Can you work these out from the model? Positions are in its coordinate system, mm. Face numbers are marked on the shaded views. Coordinates: 2 decimals unless noted, no trailing zeros. Order: outer loops, then holes, each group sorted by start corner. A loop starts at its lowest first (then second) coordinate and runs counter-clockwise, first axis right, second up. Notation, with made-up numbers: (79.5, -9) - (134.5, -9) arc R20 ccw to (134.5, 8) - close; hole circle Ø3 at (26, -7). An arc over 180 degrees is marked (long way). Use a Markdown table: item, result. Add a question column.
(1) If I drill on L1, parallel to Y at x = 0, z = 1.9; L2, parallel to X at y = -34.5, z = 1.95; L3, parallel to Y at x = 7.75, z = 0.95, over which ranges is the centre line in solid material (lowest first)? Write a range as [from, to].
(2) I want a section at D-D (x = 5.5). List the corners of the cut face in (y, z) for me.
(3) I want a section at B-B (z = 1.35). List the corners of the cut face in (x, y) for me.
(4) I want a section at C-C (y = -24.25). List the corners of the cut face in (x, z) for me, and give its area (4 significant figures).
(5) We'd pull the mould along Y, two halves only. Please class the marked faces 1, 2, 3 and 4: pulls with the +Y half, pulls with the -Y half, needs draft (parallel to the pull), parting line crosses it, or undercut.
(6) I want a section at A-A (x = 0). List the corners of the cut face in (y, z) for me, and give its area (3 significant figures).
(7) For pin 1 Ø1.5 at (y, z) = (-5, 2.5) entering from -X, with a flat end and sliding along its axis, tell me the tip position at first contact or that it passes through.
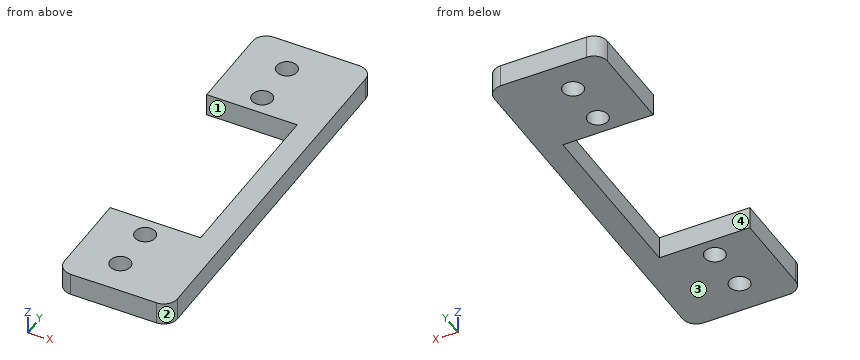
```python
from build123d import *

# Parameters (mm, degrees)
BOSS_EXTRUDE1_DEPTH  = 5
M4_CLEARANCE_HOLE1_D = 4.5
FILLET1_R            = 3
M4_CLEARANCE_HOLE2_D = 4.5


with BuildPart() as part:
    # Sketch2 → Boss-Extrude1 (new body)
    with BuildSketch(Plane.XY):
        Polygon((15, 42), (-10, 42), (-10, 20), (10, 20), (10, -20), (-10, -20), (-10, -42), (15, -42), align=None)
    extrude(amount=BOSS_EXTRUDE1_DEPTH)

    # M4 Clearance Hole1 (through all)
    with Locations(Plane(origin=(0, 0, 0), x_dir=(1, 0, 0), z_dir=(0, 0, -1))):
        with Locations((0, -34.5), (0, 34.5)):
            Hole(M4_CLEARANCE_HOLE1_D / 2)

    # Fillet1
    fillet1_edges = [part.edges().sort_by_distance(p)[0] for p in [
        (-10, 42, 2.5),
        (15, 42, 2.5),
        (15, -42, 2.5),
        (-10, -42, 2.5),
    ]]
    fillet(fillet1_edges, radius=FILLET1_R)

    # M4 Clearance Hole2 (through all)
    with Locations(Plane(origin=(0, 0, 0), x_dir=(1, 0, 0), z_dir=(0, 0, -1))):
        with Locations((0, -24.25), (0, 24.25)):
            Hole(M4_CLEARANCE_HOLE2_D / 2)


solid = part.part
```
Answers follow:
| question | item | result |
|---|---|---|
| 1 | L1 | y = [-42, -36.75], [-32.25, -26.5], [-22, -20], [20, 22], [26.5, 32.25], [36.75, 42] |
| 1 | L2 | x = [-10, -2.25], [2.25, 15] |
| 1 | L3 | y = [-42, -20], [20, 42] |
| 2 | outline | (-42, 0) - (-20, 0) - (-20, 5) - (-42, 5) - close; (20, 0) - (42, 0) - (42, 5) - (20, 5) - close |
| 3 | outline | (-10, -39) arc R3 ccw to (-7, -42) - (12, -42) arc R3 ccw to (15, -39) - (15, 39) arc R3 ccw to (12, 42) - (-7, 42) arc R3 ccw to (-10, 39) - (-10, 20) - (10, 20) - (10, -20) - (-10, -20) - close; hole circle Ø4.5 at (0, -34.5); hole circle Ø4.5 at (0, -24.25); hole circle Ø4.5 at (0, 24.25); hole circle Ø4.5 at (0, 34.5) |
| 4 | outline | (-10, 0) - (-2.25, 0) - (-2.25, 5) - (-10, 5) - close; (2.25, 0) - (15, 0) - (15, 5) - (2.25, 5) - close |
| 4 | area | 102.5 mm² |
| 5 | face 1 | undercut |
| 5 | face 2 | pulls with the -Y half |
| 5 | face 3 | needs draft |
| 5 | face 4 | undercut |
| 6 | outline | (-42, 0) - (-36.75, 0) - (-36.75, 5) - (-42, 5) - close; (-32.25, 0) - (-26.5, 0) - (-26.5, 5) - (-32.25, 5) - close; (-22, 0) - (-20, 0) - (-20, 5) - (-22, 5) - close; (20, 0) - (22, 0) - (22, 5) - (20, 5) - close; (26.5, 0) - (32.25, 0) - (32.25, 5) - (26.5, 5) - close; (36.75, 0) - (42, 0) - (42, 5) - (36.75, 5) - close |
| 6 | area | 130 mm² |
| 7 | pin 1 | stops at x = 10 |
